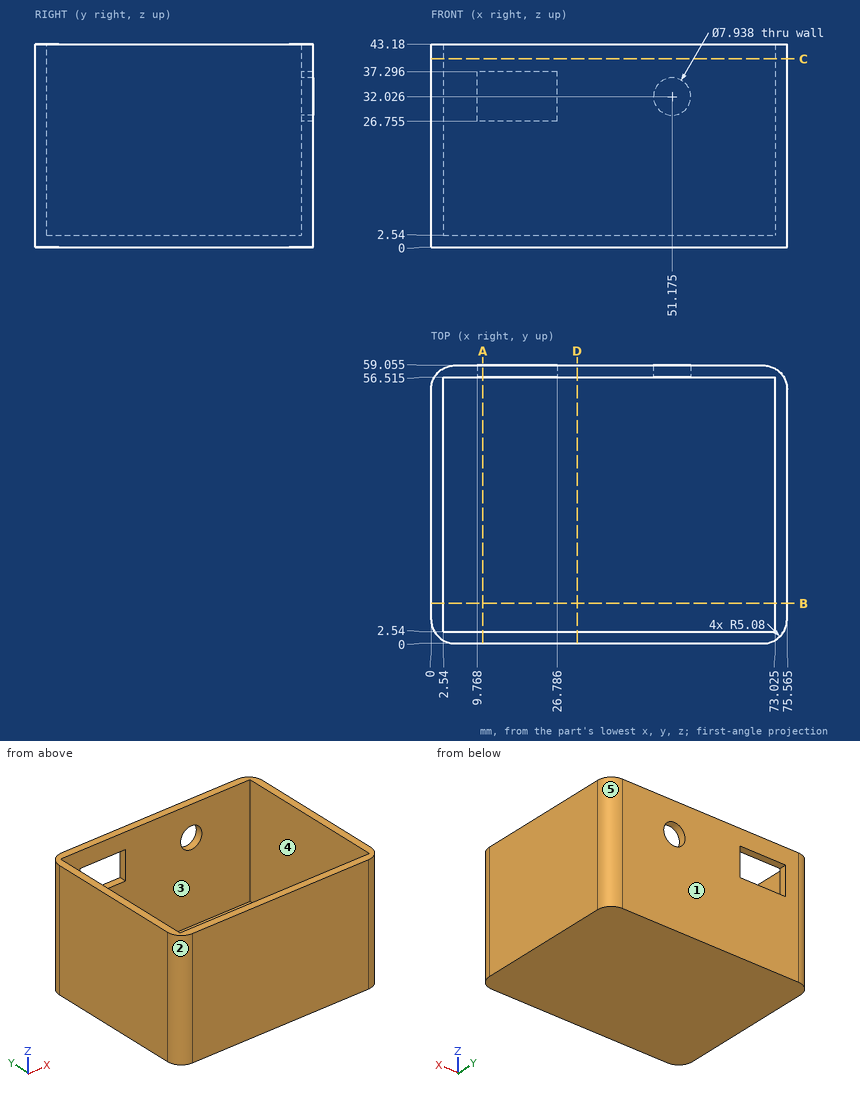
Drawing for the job (mm, zero at the part's lowest x, y, z). A direction names the side the tool comes from. Round coordinates to 2 decimals unless told otherwise and drop trailing zeros. Loops run counter-clockwise (first coordinate to the right, second up) from the corner with the lowest first, then second, coordinate; pieces in that order, holes last. Notation, with made-up numbers: (58.25, 47) -> (99.25, 47) arc R22 ccw to (99.25, 78) -> close; hole circle Ø11 at (42.25, -13). An arc over 180 degrees is marked (long way). Answer in a Markdown table with one row per item.
Item 1: Saw through at B-B (y = 8.5). Write the cut outline in (x, z) (1 decimal).
Answers below:
| item | result |
|---|---|
| outline | (0, 0) -> (75.6, 0) -> (75.6, 43.2) -> (73, 43.2) -> (73, 2.5) -> (2.5, 2.5) -> (2.5, 43.2) -> (0, 43.2) -> close |
Item 2: Pin check, flat tips, straight feed: pin 1 (1.5 mm diameter, centred on x = 34.5, y = 30.5, fed in from +Z); pin 2 (1.3 mm diameter, centred on y = 57.5, z = 34.5, fed in from -X); pin 3 (3 mm diameter, centred on y = 57.5, z = 34.5, fed in from +X) (1 decimal). Stop position of each tip, or through.
Answers below:
| item | result |
|---|---|
| pin 1 | stops at z = 2.54 |
| pin 2 | stops at x = 0.89 |
| pin 3 | stops at x = 75.1 |
Item 3: Which spindle directions (+Z, -Z, +X, -X, +Y, -Y) get a long thin tool onto all of the face, cutting with end or side? Do the marked faces 4 and 5. Say none if no direction does.
Answers below:
| item | result |
|---|---|
| face 4 | +Z |
| face 5 | +Z, -Z, +X, +Y |
Item 4: Saw through at C-C (z = 40). Write the cut outline in (x, y) (1 decimal).
Answers below:
| item | result |
|---|---|
| outline | (0, 5.1) arc R5.1 ccw to (5.1, 0) -> (70.5, 0) arc R5.1 ccw to (75.6, 5.1) -> (75.6, 54) arc R5.1 ccw to (70.5, 59.1) -> (5.1, 59.1) arc R5.1 ccw to (0, 54) -> close; hole (2.5, 2.5) -> (73, 2.5) -> (73, 56.5) -> (2.5, 56.5) -> close |
Item 5: Drill centre lines: L1, parallel to X at y = 12, z = 11 (1 decimal); L2, parallel to Y at x = 61, z = 4.5 (1 decimal); L3, parallel to Z at x = 59, y = 27.5. Where is each one in solid material? Low to high. Write a range as [from, to].
Answers below:
| item | result |
|---|---|
| L1 | x = [0, 2.5], [73, 75.6] |
| L2 | y = [0, 2.5], [56.5, 59.1] |
| L3 | z = [0, 2.54] |
Item 6: Saw through at D-D (x = 31). Write the cut outline in (y, z) (1 decimal).
Answers below:
| item | result |
|---|---|
| outline | (0, 0) -> (59.1, 0) -> (59.1, 43.2) -> (56.5, 43.2) -> (56.5, 2.5) -> (2.5, 2.5) -> (2.5, 43.2) -> (0, 43.2) -> close |
Item 7: Mould opens along X. For the marked faces 1, 2 and 3 say: +X half, -X half, draft (parallel to the pull), parting line (faces both ways), or undercut.
Answers below:
| item | result |
|---|---|
| face 1 | draft |
| face 2 | -X half |
| face 3 | undercut |
Item 8: Saw through at A-A (x = 11). Write the cut outline in (y, z) (1 decimal).
Answers below:
| item | result |
|---|---|
| outline | (0, 0) -> (59.1, 0) -> (59.1, 26.8) -> (56.5, 26.8) -> (56.5, 2.5) -> (2.5, 2.5) -> (2.5, 43.2) -> (0, 43.2) -> close; (56.5, 37.3) -> (59.1, 37.3) -> (59.1, 43.2) -> (56.5, 43.2) -> close |
